Verification items for the finished model (mm, model axes). Coordinates: 2 decimals unless noted, no trailing zeros. Write each loop counter-clockwise with the first axis right and the second up, starting at its lowest first coordinate (ties: lowest second). Pieces come first, ordered by that corner, then holes. Notation, with made-up numbers: (62, -5) -> (84, -5) arc R12 ccw to (84, 10) -> close; hole circle Ø11 at (12.5, 8.25). An arc over 180 degrees is marked (long way). Use CSV: the item, a comma, the result in double quotes.
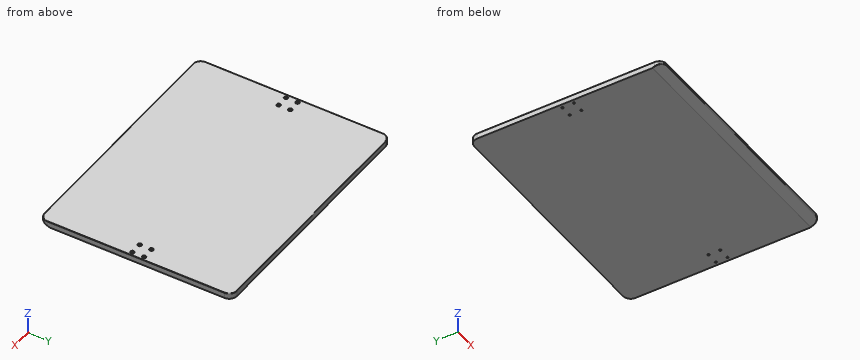
```python
from build123d import *

# Parameters (mm, degrees)
SKETCH1_W                              = 650
SKETCH1_H                              = 500
BASE_DEPTH                             = 15
COUNTERBORED_M5_BOLT_HOLES_D           = 5.5
COUNTERBORED_M5_BOLT_HOLES_CBORE_D     = 10
COUNTERBORED_M5_BOLT_HOLES_CBORE_DEPTH = 5
ROUND_CORNERS_R                        = 20
BREAK_TOP_EDGE_R                       = 1
CHAMFER2_SIZE                          = 9.099255857
CHAMFER2_SIZE_2                        = 25
FILLET3_R                              = 1


with BuildPart() as part:
    # Sketch1 → base (new body)
    with BuildSketch(Plane.XY):
        with Locations((325, 250)):
            Rectangle(SKETCH1_W, SKETCH1_H)
    extrude(amount=BASE_DEPTH)

    # counterbored M5 bolt holes (through all)
    with Locations(Plane.XY.offset(15)):
        with Locations((10, 265), (40, 235), (10, 235), (40, 265)):
            counterbored_m5_bolt_holes = CounterBoreHole(COUNTERBORED_M5_BOLT_HOLES_D / 2, COUNTERBORED_M5_BOLT_HOLES_CBORE_D / 2, COUNTERBORED_M5_BOLT_HOLES_CBORE_DEPTH)

    # mirror counterbored bolt holes: counterbored M5 bolt holes across plane
    add(counterbored_m5_bolt_holes.mirror(Plane.ZY.offset(-325)), mode=Mode.SUBTRACT)

    # round corners
    round_corners_edges = [part.edges().sort_by_distance(p)[0] for p in [
        (0, 500, 7.5),
        (650, 500, 7.5),
        (650, 0, 7.5),
        (0, 0, 7.5),
    ]]
    fillet(round_corners_edges, radius=ROUND_CORNERS_R)

    # break top edge
    break_top_edge_edges = [part.edges().sort_by_distance(p)[0] for p in [
        (0, 250, 15),
        (325, 500, 15),
        (325, 0, 15),
        (650, 250, 15),
        (5.857864376, 5.857864376, 15),
        (644.142135624, 5.857864376, 15),
        (644.142135624, 494.142135624, 15),
        (5.857864376, 494.142135624, 15),
    ]]
    fillet(break_top_edge_edges, radius=BREAK_TOP_EDGE_R)

    # Chamfer2
    # the kernel refuses this chamfer: 25, 9.099255857 mm, written as the material it takes off along each edge
    with BuildSketch(Plane(origin=(-44.854868314, 0, 0), x_dir=(0, -0.09904090225204935, 0.9950833631817486), z_dir=(1, 0, 0))) as chamfer2_piece_1:
        Polygon((CHAMFER2_SIZE * 0.995083363144, -CHAMFER2_SIZE * 0.0990409022483), (-CHAMFER2_SIZE_2 * 0.099040902252, -CHAMFER2_SIZE_2 * 0.995083363182), (0, 0), align=None)
    extrude(amount=739.709736628, mode=Mode.SUBTRACT)

    # Fillet3
    fillet3_edges = [part.edges().sort_by_distance(p)[0] for p in [
        (325, 0, 9.099255857),
        (644.360022397, 6.079161061, 6.886622181),
        (650, 22.5, 0.909925586),
        (325, 25, 0),
        (0, 22.5, 0.909925586),
        (5.639977603, 6.079161061, 6.886622181),
    ]]
    fillet(fillet3_edges, radius=FILLET3_R)


solid = part.part
```
1) Cross-section at B-B (z = 5.75). Give the number of separate pieces and of enclosed holes in the cut face, plus the area to 3 significant figures.
Return value:
separate pieces,"1"
enclosed holes,"8"
area,"319,000 mm2"
2) Scan lines: L1, parallel to X at y = 265, z = 5; L2, parallel to X at y = 265, z = 11.35; L3, parallel to X at y = 244.5, z = 14.5. Record each from-to range of solid material in increasing order.
Return value:
L1,"0 to 7.25, 12.75 to 37.25, 42.75 to 607.25, 612.75 to 637.25, 642.75 to 650"
L2,"0 to 5, 15 to 35, 45 to 605, 615 to 635, 645 to 650"
L3,"0.13 to 649.87"
3) Cross-section at A-A (x = 465.5). Record the boundary of the cut face in (y, z), plus the area to 3 significant figures.
Return value:
outline,"(0, 9.8) arc R1 ccw to (0.66, 8.86) -> (24.83, 0.06) arc R1 ccw to (25.18, 0) -> (500, 0) -> (500, 14) arc R1 ccw to (499, 15) -> (1, 15) arc R1 ccw to (0, 14) -> close"
area,"7,390 mm2"
4) Gauge pin test, flat ends, axial feed: pin 1 (6.5 mm diameter, centred on x = 640, y = 235, fed in from -Z); pin 2 (7 mm diameter, centred on x = 40, y = 265, fed in from +Z). Record the tip position at first contact, or that the pin passes through.
Return value:
pin 1,"z = 0"
pin 2,"z = 10"
